Here's how the part is built. I have some questions about the finished solid (model axes, mm). A direction names the side the tool comes from. Round coordinates to 2 decimals unless told otherwise and drop trailing zeros. Write each loop counter-clockwise with the first axis right and the second up, starting at its lowest first coordinate (ties: lowest second). Pieces come first, ordered by that corner, then holes. Notation, with made-up numbers: (-39.5, 32) -> (-1.5, 32) arc R15 cw to (-1.5, 49) -> close; hole circle Ø6 at (45, -34). An arc over 180 degrees is marked (long way). Put each result on its own line as item: value. Start each with the question number.
1. Suppose I cut it at A-A (y = -5). Please give me the cut outline in (x, z).
2. Which directions (+Z, -Z, +X, -X, +Y, -Y) give clear straight access to the entire face, cutting with the end or side of a thin tool? Please do faces 1 (the face through (3.04, -25.85, 16.61)), 2 (the face through (5.14, 1.97, -32.1)), 3 (the face through (3, -14, 21.75)), 4 (the face through (3, 0, -28)).
3. Suppose I cut it at C-C (z = -19.5). Please give me the cut outline in (x, y), then the cut area to 3 significant figures.
4. For pin 1 (1.8 mm diameter, centred on x = 4, y = -18.5, fed in from -Z); pin 2 (3 mm diameter, centred on y = -5, z = 18.75, fed in from -X); pin 3 (1.5 mm diameter, centred on x = 4, y = -7, fed in from +Z); pin 4 (1.8 mm diameter, centred on x = 4, z = 1, fed in from -Y), each with a flat end and sliding along its axis, tell me the tip position at first contact or that it passes through.
5. I need wall thicknesses on probe 1 along Y at (x, z) = (3.45, 18.75); probe 2 along Z at (x, y) = (3, 1.7); probe 3 along Z at (x, y) = (4.15, -13). Which ranges of each line are inside material? Lowest first, please. Write a range as from..to.
6. Suppose I cut it at B-B (y = 1). Count the separate pieces of the cut face and the enclosed holes in it, then the cut area to 3 significant figures.
7. We'd pull the mould along Y, two halves only. Please class faces 5 (the face through (3, -4.3, 20.3)), 6 (the face through (3.04, -25.85, -20.89)), 7 (the face through (2.958, -25.183, 19.664)), 8 (the face through (3, -13, 15.75)): +Y half, -Y half, draft (parallel to the pull), parting line (faces both ways), or undercut.
```python
from build123d import *

# Parameters (mm, degrees)
SKETCH1_R                                       = 1.7
BOSS_EXTRUDE1_DEPTH                             = 6
CSK_FOR_M3_FLAT_HEAD_MACHINE_SCREW1_D           = 3.4
CSK_FOR_M3_FLAT_HEAD_MACHINE_SCREW1_DEPTH       = 6
CSK_FOR_M3_FLAT_HEAD_MACHINE_SCREW1_CSINK_D     = 3.5
CSK_FOR_M3_FLAT_HEAD_MACHINE_SCREW1_CSINK_ANGLE = 90
CSK_FOR_M3_FLAT_HEAD_MACHINE_SCREW1_TIP         = 1.021463052
FILLET1_R                                       = 3
FILLET2_R                                       = 3
FILLET3_R                                       = 3


with BuildPart() as part:
    # Sketch1 → Boss-Extrude1 (new body)
    with BuildSketch(Plane(origin=(0, 0, 0), x_dir=(0, 0, -1), z_dir=(1, 0, 0))):
        Polygon((-21.75, -26.75), (-21.75, 0), (-33, 0), (-33, 4), (33, 4), (33, 0), (21.75, 0), (21.75, -26.75), (15.75, -26.75), (15.75, 0), (-15.75, 0), (-15.75, -26.75), align=None)
        with Locations((18.75, -5)):
            Circle(SKETCH1_R, mode=Mode.SUBTRACT)
        with Locations((18.75, -23.75)):
            Circle(SKETCH1_R, mode=Mode.SUBTRACT)
        with Locations(Location((-18.75, -23.75, 0), (0, 0, 180))):
            Circle(SKETCH1_R, mode=Mode.SUBTRACT)
        with Locations(Location((-18.75, -5, 0), (0, 0, 180))):
            Circle(SKETCH1_R, mode=Mode.SUBTRACT)
    extrude(amount=BOSS_EXTRUDE1_DEPTH)

    # CSK for M3 Flat Head Machine Screw1
    with Locations(Plane(origin=(0, 4, 0), x_dir=(1, 0, 0), z_dir=(0, 1, 0))):
        with Locations((3, 30), (3, -30)):
            CounterSinkHole(CSK_FOR_M3_FLAT_HEAD_MACHINE_SCREW1_D / 2, CSK_FOR_M3_FLAT_HEAD_MACHINE_SCREW1_CSINK_D / 2, depth=CSK_FOR_M3_FLAT_HEAD_MACHINE_SCREW1_DEPTH, counter_sink_angle=CSK_FOR_M3_FLAT_HEAD_MACHINE_SCREW1_CSINK_ANGLE)
            with Locations((0, 0, -(CSK_FOR_M3_FLAT_HEAD_MACHINE_SCREW1_DEPTH + CSK_FOR_M3_FLAT_HEAD_MACHINE_SCREW1_TIP / 2))):  # 118° drill point
                Cone(0, CSK_FOR_M3_FLAT_HEAD_MACHINE_SCREW1_D / 2, CSK_FOR_M3_FLAT_HEAD_MACHINE_SCREW1_TIP, mode=Mode.SUBTRACT)

    # Fillet1
    fillet1_edges = [part.edges().sort_by_distance(p)[0] for p in [
        (3, -26.75, -21.75),
        (3, -26.75, -15.75),
        (3, -26.75, 15.75),
        (3, -26.75, 21.75),
    ]]
    fillet(fillet1_edges, radius=FILLET1_R - 0.0001)  # a hair under: the kernel refuses the full size

    # Fillet2
    fillet2_edges = [part.edges().sort_by_distance(p)[0] for p in [
        (3, 0, 21.75),
        (3, 0, -21.75),
        (3, 0, -15.75),
        (3, 0, 15.75),
    ]]
    fillet(fillet2_edges, radius=FILLET2_R)

    # Fillet3
    fillet3_edges = [part.edges().sort_by_distance(p)[0] for p in [
        (6, 2, -33),
        (0, 2, -33),
        (0, 2, 33),
        (6, 2, 33),
    ]]
    fillet(fillet3_edges, radius=FILLET3_R - 0.0001)  # a hair under: the kernel refuses the full size


solid = part.part
```
Verdict:
1. outline: (0, -21.75) -> (6, -21.75) -> (6, -20.45) -> (0, -20.45) -> close; (0, -17.05) -> (6, -17.05) -> (6, -15.75) -> (0, -15.75) -> close; (0, 15.75) -> (6, 15.75) -> (6, 17.05) -> (0, 17.05) -> close; (0, 20.45) -> (6, 20.45) -> (6, 21.75) -> (0, 21.75) -> close
2. face 1: +X, -X, -Y
2. face 2: -Z, +X, +Y, -Y
2. face 3: +Z, +X, -X, -Y
2. face 4: -Z, +X, -X, -Y
3. outline: (0, -26.65) -> (6, -26.65) -> (6, -25.28) -> (0, -25.28) -> close; (0, -22.22) -> (6, -22.22) -> (6, -6.53) -> (0, -6.53) -> close; (0, -3.47) -> (6, -3.47) -> (6, 4) -> (0, 4) -> close
3. area: 147 mm^2
4. pin 1: stops at z = -21.75
4. pin 2: passes through
4. pin 3: stops at z = 21.75
4. pin 4: stops at y = 0
5. probe 1: y = -26.75..-25.45, -22.05..-6.7, -3.3..4
5. probe 2: z = -33..-31.7, -28.3..28.3, 31.7..33
5. probe 3: z = -21.75..-15.75, 15.75..21.75
6. separate pieces: 1
6. enclosed holes: 2
6. area: 370 mm^2
7. face 5: undercut
7. face 6: -Y half
7. face 7: undercut
7. face 8: draft
